Design review of the part built by this model. Coordinates are the model's own, in mm. Coordinates: 2 decimals unless noted, no trailing zeros. Write each loop counter-clockwise with the first axis right and the second up, starting at its lowest first coordinate (ties: lowest second). Pieces come first, ordered by that corner, then holes. Notation, with made-up numbers: M 50,51 L 88,51 A37 ccw 88,90 Z; hole C -10.75,11.5 d2. An arc over 180 degrees is marked long. Write item = value, one per line.
```python
from build123d import *

# Parameters (mm, degrees)
SKETCH_2_W          = 46
SKETCH_2_H          = 46
SKETCH_2_R          = 18
EXTRUDE_1_DEPTH     = 5
FILLET_1_R          = 5.5
SKETCH_3_R          = 1.6
CUT_EXTRUDE_1_DEPTH = 33.908965344
SKETCH_4_R          = 65
SKETCH_4_R_2        = 1.6
SKETCH_4_R_3        = 18
EXTRUDE_2_DEPTH     = 5
SKETCH_7_R          = 1.6
CUT_EXTRUDE_3_DEPTH = 93.059763198


with BuildPart() as part:
    # 草图2 → 凸台-拉伸1 (new body)
    with BuildSketch(Plane(origin=(0, 0, 0), x_dir=(1, 0, 0), z_dir=(0, 1, 0))):
        Rectangle(SKETCH_2_W, SKETCH_2_H)
        with Locations(Location((0, 0, 0), (0, 0, 270))):
            Circle(SKETCH_2_R, mode=Mode.SUBTRACT)
    extrude(amount=EXTRUDE_1_DEPTH)

    # 圆角1
    fillet_1_edges = [part.edges().sort_by_distance(p)[0] for p in [
        (23, 2.5, 23),
        (-23, 2.5, 23),
        (-23, 2.5, -23),
        (23, 2.5, -23),
    ]]
    fillet(fillet_1_edges, radius=FILLET_1_R)

    # 草图3 → 切除-拉伸1 (cut, through all)
    with BuildSketch(Plane(origin=(0, 5, 0), x_dir=(1, 0, 0), z_dir=(0, 1, 0))):
        with Locations(Location((-15.5, 15.5, 0), (0, 0, 270))):
            Circle(SKETCH_3_R)
        with Locations(Location((15.5, 15.5, 0), (0, 0, 270))):
            Circle(SKETCH_3_R)
        with Locations(Location((-15.5, -15.5, 0), (0, 0, 270))):
            Circle(SKETCH_3_R)
        with Locations(Location((15.5, -15.5, 0), (0, 0, 270))):
            Circle(SKETCH_3_R)
    extrude(amount=-CUT_EXTRUDE_1_DEPTH, mode=Mode.SUBTRACT)

    # 草图4 → 凸台-拉伸2 (add)
    # profile 1 of 2: a face of its own
    with BuildSketch(Plane(origin=(0, 5, 0), x_dir=(1, 0, 0), z_dir=(0, 1, 0))):
        with Locations(Location((0, 0, 0), (0, 0, 270))):
            Circle(SKETCH_4_R)
        with Locations(Location((-49.1, 0, 0), (0, 0, 270))):
            Circle(SKETCH_4_R_2, mode=Mode.SUBTRACT)
        with Locations(Location((0, -49.1, 0), (0, 0, 270))):
            Circle(SKETCH_4_R_2, mode=Mode.SUBTRACT)
        with Locations(Location((49.1, 0, 0), (0, 0, 270))):
            Circle(SKETCH_4_R_2, mode=Mode.SUBTRACT)
        with Locations(Location((0, 49.1, 0), (0, 0, 270))):
            Circle(SKETCH_4_R_2, mode=Mode.SUBTRACT)
        with BuildLine():
            Line((-17.5, -23), (17.5, -23))
            ThreePointArc((17.5, -23), (21.389087297, -21.389087297), (23, -17.5))
            Line((23, -17.5), (23, 17.5))
            ThreePointArc((23, 17.5), (21.389087297, 21.389087297), (17.5, 23))
            Line((17.5, 23), (-17.5, 23))
            ThreePointArc((-17.5, 23), (-21.389087297, 21.389087297), (-23, 17.5))
            Line((-23, 17.5), (-23, -17.5))
            ThreePointArc((-23, -17.5), (-21.389087297, -21.389087297), (-17.5, -23))
        make_face(mode=Mode.SUBTRACT)
    # profile 2 of 2: a face of its own
    with BuildSketch(Plane(origin=(0, 5, 0), x_dir=(1, 0, 0), z_dir=(0, 1, 0))):
        with BuildLine():
            ThreePointArc((-23, -17.5), (-21.389087297, -21.389087297), (-17.5, -23))
            Line((-17.5, -23), (17.5, -23))
            ThreePointArc((17.5, -23), (21.389087297, -21.389087297), (23, -17.5))
            Line((23, -17.5), (23, 17.5))
            ThreePointArc((23, 17.5), (21.389087297, 21.389087297), (17.5, 23))
            Line((17.5, 23), (-17.5, 23))
            ThreePointArc((-17.5, 23), (-21.389087297, 21.389087297), (-23, 17.5))
            Line((-23, 17.5), (-23, -17.5))
        make_face()
        with Locations(Location((15.5, 15.5, 0), (0, 0, 270))):
            Circle(SKETCH_4_R_2, mode=Mode.SUBTRACT)
        with Locations(Location((-15.5, -15.5, 0), (0, 0, 270))):
            Circle(SKETCH_4_R_2, mode=Mode.SUBTRACT)
        with Locations(Location((0, 0, 0), (0, 0, 270))):
            Circle(SKETCH_4_R_3, mode=Mode.SUBTRACT)
        with Locations(Location((-15.5, 15.5, 0), (0, 0, 270))):
            Circle(SKETCH_4_R_2, mode=Mode.SUBTRACT)
        with Locations(Location((15.5, -15.5, 0), (0, 0, 270))):
            Circle(SKETCH_4_R_2, mode=Mode.SUBTRACT)
    extrude(amount=-EXTRUDE_2_DEPTH)

    # 草图7 → 切除-拉伸3 (cut, through all)
    with BuildSketch(Plane(origin=(0, 5, 0), x_dir=(1, 0, 0), z_dir=(0, 1, 0))):
        with Locations(Location((-14.383356955, 26.682742705, 0), (0, 0, 270))):
            Circle(SKETCH_7_R)
        with Locations(Location((-27.616643045, 12.496829297, 0), (0, 0, 270))):
            Circle(SKETCH_7_R)
    extrude(amount=-CUT_EXTRUDE_3_DEPTH, mode=Mode.SUBTRACT)


solid = part.part
```
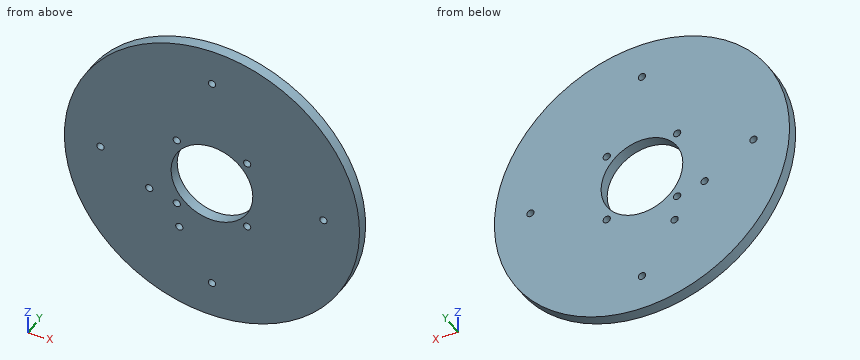
Q1. Consider section C-C, the plane z = 49.1. State the section outline as (x, y) points.
Check result:
outline = M -42.59,0 L -1.6,0 L -1.6,5 L -42.59,5 Z; M 1.6,0 L 42.59,0 L 42.59,5 L 1.6,5 Z
Q2. Wall thickness on line 1 (X direction, y = 2.7, z = 0); line 2 (Z direction, x = 16, y = 0.4); line 3 (Z direction, x = -12, y = 0.7): over which ranges is each line inside the solid? List them lowest first.
Check result:
line_1 = -65 to -50.7, -47.5 to -18, 18 to 47.5, 50.7 to 65
line_2 = -63 to -17.02, -13.98 to -8.25, 8.25 to 13.98, 17.02 to 63
line_3 = -63.88 to -13.42, 13.42 to 63.88
Q3. Consider section A-A, the plane z = 0. State the section outline as (x, y) points.
Check result:
outline = M -65,0 L -50.7,0 L -50.7,5 L -65,5 Z; M -47.5,0 L -18,0 L -18,5 L -47.5,5 Z; M 18,0 L 47.5,0 L 47.5,5 L 18,5 Z; M 50.7,0 L 65,0 L 65,5 L 50.7,5 Z
Q4. Consider section B-B, the plane x = 0. State the section outline as (y, z) points.
Check result:
outline = M 0,-65 L 5,-65 L 5,-50.7 L 0,-50.7 Z; M 0,-47.5 L 5,-47.5 L 5,-18 L 0,-18 Z; M 0,18 L 5,18 L 5,47.5 L 0,47.5 Z; M 0,50.7 L 5,50.7 L 5,65 L 0,65 Z
Q5. Consider section D-D, the plane x = -49.1. State the section outline as (y, z) points.
Check result:
outline = M 0,-42.59 L 5,-42.59 L 5,-1.6 L 0,-1.6 Z; M 0,1.6 L 5,1.6 L 5,42.59 L 0,42.59 Z
Q6. For P1, Ø1, axis at x = 6.5, y = 1.5, coming from the +Z side; P2, Ø3, axis at x = -12.5, y = 1, coming from the +Z side; P3, Ø1.5, axis at x = -30.5, y = 4, coming from the -Z side, all flat-tipped, find the tip position at first contact; note any pin that passes through.
Check result:
P1 = 64.72
P2 = 64.06
P3 = -57.79
